Can you work these out from the drawing? Everything is in mm from the part's minimum corner. Round coordinates to 2 decimals unless told otherwise and drop trailing zeros. Write each loop counter-clockwise with the first axis right and the second up, starting at its lowest first coordinate (ties: lowest second). Pieces come first, ordered by that corner, then holes. Notation, with made-up numbers: (24, 35.25) -> (65, 35.25) arc R25 cw to (65, 52.25) -> close; hole circle Ø4 at (23, 12). An arc over 180 degrees is marked (long way). Answer as CSV lines item,"result". Start each with the question number.
Q1. Imagine slicing it at D-D on z = 35.5. Please give me the cut outline in (x, y), and give its area (3 significant figures).
Q2. If I drill on line 1 (Z direction, x = 129, y = 16); line 2 (Z direction, x = 113, y = 72); line 3 (X direction, y = 47.5, z = 178.5), over which ranges is the centre line in solid material (lowest first)? Write a range as [from, to].
Q3. Imagine slicing it at B-B on x = 57. Please give me the cut outline in (y, z), and give its area (3 significant figures).
Q4. Imagine slicing it at A-A on z = 98.5. Please give me the cut outline in (x, y), and give its area (3 significant figures).
Q5. If we mould it in two halves opening along Z, with no side actions, what happens to the marked faces 1, 2, 3 and 4? For each: pulls with the +Z half, pulls with the -Z half, needs draft (parallel to the pull), parting line crosses it, or undercut.
Q6. Imagine slicing it at C-C on y = 40. Please give me the cut outline in (x, z), and give its area (3 significant figures).
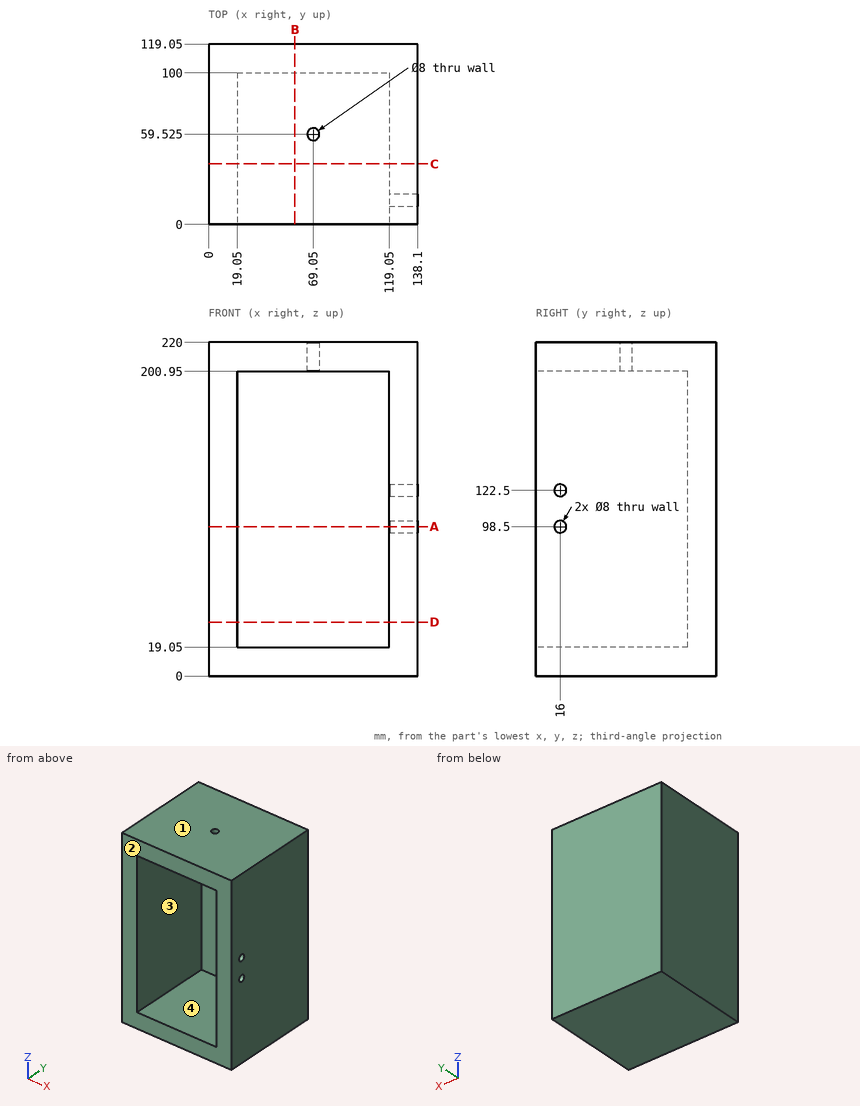
Checks:
1,outline,"(0, 0) -> (19.05, 0) -> (19.05, 100) -> (119.05, 100) -> (119.05, 0) -> (138.1, 0) -> (138.1, 119.05) -> (0, 119.05) -> close"
1,area,"6,440 mm^2"
2,line 1,"[0, 94.5], [102.5, 118.5], [126.5, 220]"
2,line 2,"[0, 19.05], [200.95, 220]"
2,line 3,"[0, 19.05], [119.05, 138.1]"
3,outline,"(0, 0) -> (119.05, 0) -> (119.05, 220) -> (0, 220) -> (0, 200.95) -> (100, 200.95) -> (100, 19.05) -> (0, 19.05) -> close"
3,area,"8,000 mm^2"
4,outline,"(0, 0) -> (19.05, 0) -> (19.05, 100) -> (119.05, 100) -> (119.05, 20) -> (138.1, 20) -> (138.1, 119.05) -> (0, 119.05) -> close; (119.05, 0) -> (138.1, 0) -> (138.1, 12) -> (119.05, 12) -> close"
4,area,"6,290 mm^2"
5,face 1,"pulls with the +Z half"
5,face 2,"needs draft"
5,face 3,"undercut"
5,face 4,"undercut"
6,outline,"(0, 0) -> (138.1, 0) -> (138.1, 220) -> (0, 220) -> close; hole (19.05, 19.05) -> (119.05, 19.05) -> (119.05, 200.95) -> (19.05, 200.95) -> close"
6,area,"12,200 mm^2"
